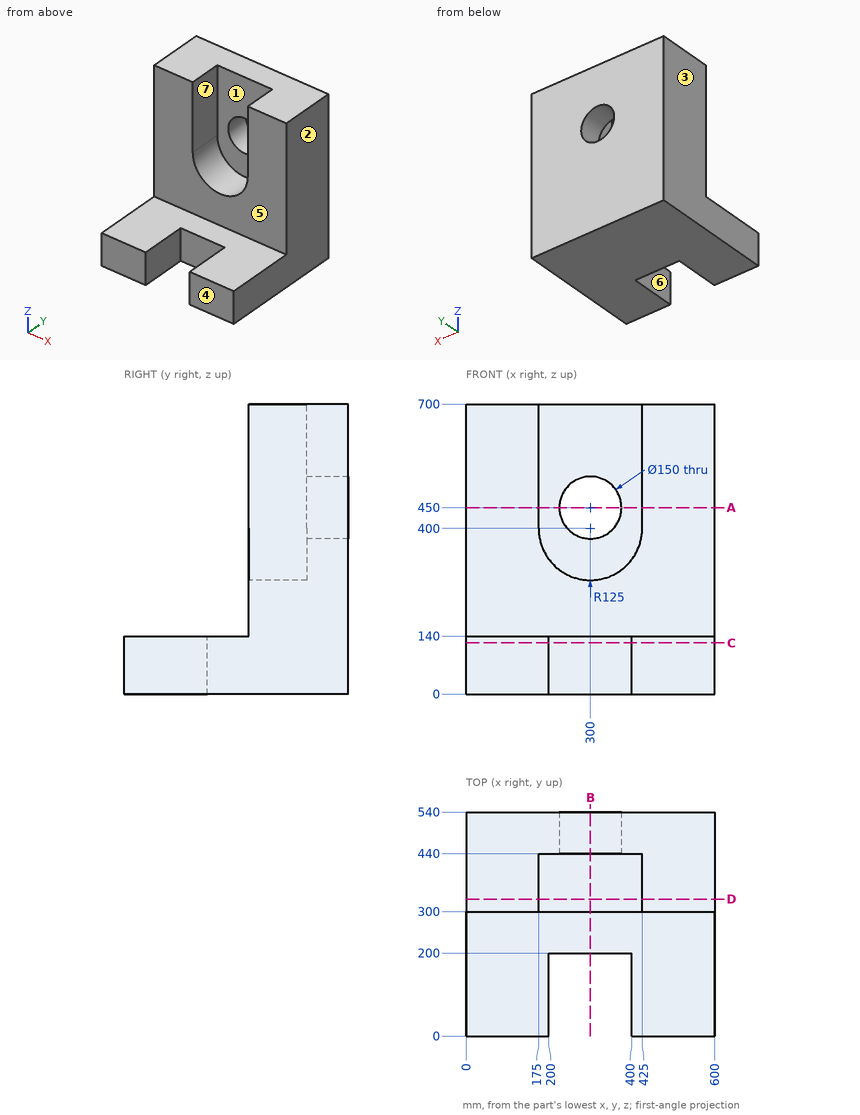
Drawing for the job (mm, zero at the part's lowest x, y, z). A direction names the side the tool comes from. Give positions to 0.01 mm unless a question says otherwise; leave off trailing zeros. Write each loop counter-clockwise with the first axis right and the second up, starting at its lowest first coordinate (ties: lowest second). Pieces come first, ordered by that corner, then holes. Notation, with made-up numbers: (78, -23) -> (121, -23) arc R22 ccw to (121, -11) -> close; hole circle Ø9 at (15, 72.5). An arc over 180 degrees is marked (long way). Put each result on its own line as item: value. Start each with the question number.
Item 1: Which spindle directions (+Z, -Z, +X, -X, +Y, -Y) get a long thin tool onto all of the face, cutting with end or side? Do the marked faces 5, 6 and 7. Say none if no direction does.
Item 2: Cut at D-D (y = 330.5). List the corners of the cut face in (x, z).
Item 3: Cut at B-B (x = 300). List the corners of the cut face in (y, z).
Item 4: Cut at A-A (z = 450). List the corners of the cut face in (x, y), then the cut area to 3 significant figures.
Item 5: Pull direction X, two halves, no side cores. Call the marked faces 1, 2, 3 and 4: pulls with the +X half, pulls with the -X half, needs draft (parallel to the pull), parting line crosses it, or undercut.
Item 6: Cut at C-C (z = 124). List the corners of the cut face in (x, y).
Item 7: Wall check: L1, parallel to X at y = 128.5, z = 99; L2, parallel to Z at x = 300, y = 509; L3, parallel to Y at x = 379, z = 594. Give the ranges that are in metal, low to high. Write a range as [from, to].
Item 8: Pin check, flat tips, straight feed: pin 1 Ø1 at (x, y) = (106.5, 78) entering from +Z; pin 2 Ø8 at (x, z) = (179.5, 295.5) entering from -Y. Stop position of each tip, or through.
Answer list:
1. face 5: +Z, +X, -X, -Y
1. face 6: +Z, -Z, -Y
1. face 7: +Z, -Y
2. outline: (0, 0) -> (600, 0) -> (600, 700) -> (425, 700) -> (425, 400) arc R125 cw to (175, 400) -> (175, 700) -> (0, 700) -> close
3. outline: (200, 0) -> (540, 0) -> (540, 375) -> (440, 375) -> (440, 275) -> (300, 275) -> (300, 140) -> (200, 140) -> close; (440, 525) -> (540, 525) -> (540, 700) -> (440, 700) -> close
4. outline: (0, 300) -> (175, 300) -> (175, 440) -> (225, 440) -> (225, 540) -> (0, 540) -> close; (375, 440) -> (425, 440) -> (425, 300) -> (600, 300) -> (600, 540) -> (375, 540) -> close
4. area: 94,000 mm2
5. face 1: undercut
5. face 2: pulls with the +X half
5. face 3: pulls with the -X half
5. face 4: needs draft
6. outline: (0, 0) -> (200, 0) -> (200, 200) -> (400, 200) -> (400, 0) -> (600, 0) -> (600, 540) -> (0, 540) -> close
7. L1: x = [0, 200], [400, 600]
7. L2: z = [0, 375], [525, 700]
7. L3: y = [440, 540]
8. pin 1: stops at z = 140
8. pin 2: stops at y = 300
